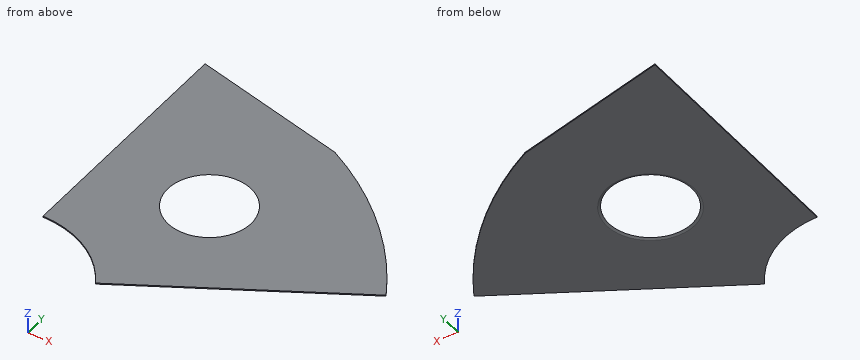
Solid Edge part; units mm, degrees
sketch "Sketch1" plane through (0, 0, 0) normal (0, 0, 1) x (1, 0, 0)
  line L0 (483.7062, 279.7959) -> (1671.5468, 965.5959)
  arc A0 (483.7062, 279.7959) -> (0.4572, 558.7998) centre (0, 0) ccw
  line L1 (0.4572, 558.7998) -> (0.4572, 1930.2902)
  line L2 (0.4572, 1930.2902) -> (876.4259, 1719.9773)
  arc A1 (876.4259, 1719.9773) -> (1671.5468, 965.5959) centre (0, 0) cw
extrude "Protrusion1" add sketch "Sketch1" against normal blind 6.35
sketch "Sketch2" plane through (610.0572, 1056.6501, 0) normal (0.5, 0.866, 0) x (-0.866, 0.5, 0)
  arc A0 (0, 50.8) -> (571.5, -520.7) centre (0, -520.7) cw
  line L0 (571.5, -520.7) -> (0, -520.7)
  line L1 (0, -520.7) -> (0, 50.8)
revolve "RevolvedCutout1" cut sketch "Sketch2" angle 360 about axis through (610.0572, 1056.6501, 0) along (0, 0, -1)
Can you work these out from the model? Positions are in its coordinate system, mm. Round coordinates to 2 decimals unless told otherwise and drop trailing zeros. Loops run counter-clockwise (first coordinate to the right, second up) from the corner with the lowest first, then second, coordinate; pieces in that order, holes last. Notation, with made-up numbers: (22.25, -34) -> (60.25, -34) arc R19 ccw to (60.25, -18) -> close; hole circle Ø3 at (-12.75, 17). An arc over 180 degrees is marked (long way). One line per item, written item: value. Start each with the question number.
1. If we section it at A-A, the plane y = 901.5: Write out the boundary of the cut face in (x, z).
2. If I drill on probe 1 along X at (y, z) = (1041, -4); probe 2 along Y at (x, z) = (708, -4.25); probe 3 along Y at (x, z) = (1166, -2.25), over which ranges is the centre line in solid material (lowest first)?
3. For pin 1 (1 mm diameter, centred on x = 1014, z = -4, fed in from +Y), with a flat end and sliding along its axis, tell me the tip position at first contact or that it passes through.
4. If we section it at C-C, the plane z = -3: Write out the boundary of the cut face in (x, y).
5. If we section it at D-D, the plane y = 1636.5: Write out the boundary of the cut face in (x, z), then the cut area to 3 significant figures.
6. If we section it at B-B, the plane x = 520: Write out the boundary of the cut face in (y, z), then the cut area to 3 significant figures.
Calculated:
1. outline: (0.46, -6.35) -> (415.16, -6.35) arc R550.04 cw to (432.82, 0) -> (0.46, 0) -> close; (787.29, 0) arc R550.04 cw to (804.95, -6.35) -> (1560.53, -6.35) -> (1560.53, 0) -> close
2. probe 1: x = 0.46 to 366.36, 853.75 to 1625.66
2. probe 2: y = 409.29 to 832.38, 1280.92 to 1760.41
2. probe 3: y = 673.72 to 1538.47
3. pin 1: stops at y = 1642.94
4. outline: (0.46, 558.8) arc R558.8 cw to (483.71, 279.8) -> (1671.55, 965.6) arc R1930.4 ccw to (876.43, 1719.98) -> (0.46, 1930.29) -> close; hole circle Ø484.14 at (610.06, 1056.65)
5. outline: (0.46, -6.35) -> (1023.87, -6.35) -> (1023.87, 0) -> (0.46, 0) -> close
5. area: 6,500 mm²
6. outline: (300.75, -6.35) -> (824.39, -6.35) arc R564.36 cw to (839, 0) -> (300.75, 0) -> close; (1274.3, 0) arc R564.36 cw to (1288.91, -6.35) -> (1805.55, -6.35) -> (1805.55, 0) -> close
6. area: 6,700 mm²
